```python
from build123d import *

# Parameters (mm, degrees)
PAD_DEPTH       = 15
SKETCH001_W     = 60
SKETCH001_H     = 15
PAD001_DEPTH    = 5
SKETCH002_W     = 60
SKETCH002_H     = 15
PAD002_DEPTH    = 5
FILLET_R        = 7
SKETCH003_W     = 3
SKETCH003_H     = 15
PAD003_DEPTH    = 3
CHAMFER_SIZE    = 2
SKETCH004_R     = 3.25
POCKET_DEPTH    = 60.001
POCKET001_DEPTH = 33
FILLET001_R     = 2


with BuildPart() as part:
    # Sketch → Pad (new body)
    with BuildSketch(Plane.XY):
        Polygon((0, 0), (30, 0), (30, 15), (-15, 15), align=None)
    extrude(amount=PAD_DEPTH)

    # Sketch001 (on Face6 of Pad) → Pad001 (join)
    with BuildSketch(Plane.XY.offset(15)):
        with Locations((0, 7.5)):
            Rectangle(SKETCH001_W, SKETCH001_H)
    extrude(amount=PAD001_DEPTH)

    # Sketch002 (on Face4 of Pad001) → Pad002 (join)
    with BuildSketch(Plane(origin=(0, 0, 0), x_dir=(1, 0, 0), z_dir=(0, 0, -1))):
        with Locations((0, -7.5)):
            Rectangle(SKETCH002_W, SKETCH002_H)
    extrude(amount=PAD002_DEPTH)

    # Fillet
    fillet_edges = [part.edges().sort_by_distance(p)[0] for p in [
        (-7.5, 7.5, 0),
        (-7.5, 7.5, 15),
    ]]
    fillet(fillet_edges, radius=FILLET_R)

    # Sketch003 (on Face9 of Fillet) → Pad003 (join)
    with BuildSketch(Plane.XY):
        with Locations((-28.5, 7.5)):
            Rectangle(SKETCH003_W, SKETCH003_H)
    extrude(amount=PAD003_DEPTH)

    # Chamfer
    chamfer_edges = [part.edges().sort_by_distance(p)[0] for p in [
        (-27, 7.5, 3),
    ]]
    chamfer(chamfer_edges, length=CHAMFER_SIZE)

    # Sketch004 (on Face18 of Chamfer) → Pocket (cut, through all)
    with BuildSketch(Plane.YZ.offset(30)):
        with Locations((7.5, 7.5)):
            Circle(SKETCH004_R)
    extrude(amount=-POCKET_DEPTH, mode=Mode.SUBTRACT)

    # Sketch005 (on Face23 of Pocket) → Pocket001 (cut)
    with BuildSketch(Plane(origin=(-30, 0, 0), x_dir=(0, -1, 0), z_dir=(-1, 0, 0))):
        Polygon((-7.5, 13.562178), (-12.75, 10.531089), (-12.75, 4.468911), (-7.5, 1.437822), (-2.25, 4.468911), (-2.25, 10.531089), align=None)
    extrude(amount=-POCKET001_DEPTH, mode=Mode.SUBTRACT)

    # Fillet001
    fillet001_edges = [part.edges().sort_by_distance(p)[0] for p in [
        (30, 7.5, 20),
        (30, 7.5, -5),
        (0, 0, 20),
        (0, 0, -5),
        (0, 15, 20),
        (0, 15, -5),
    ]]
    fillet(fillet001_edges, radius=FILLET001_R)


solid = part.part
```
Here's how the part is built. I have some questions about the finished solid (model axes, mm). A direction names the side the tool comes from. Give positions to 0.01 mm unless a question says otherwise; leave off trailing zeros. Order: outer loops, then holes, each group sorted by start corner. A loop starts at its lowest first (then second) coordinate and runs counter-clockwise, first axis right, second up. Notation, with made-up numbers: (71.5, 89.25) - (95.5, 89.25) arc R34 cw to (95.5, 121.25) - close; hole circle Ø6 at (78.5, 83.25). An arc over 180 degrees is marked (long way). Answer as a JSON object with one key per item and string values. Group by question number.
Item 1: For P1, Ø3, axis at y = 9.5, z = 9, coming from the -X side, with a flat end and sliding along its axis, tell me the tip position at first contact or that it passes through.
Item 2: If we section it at A-A on z = 5.25: Please give me the cut outline in (x, y).
Item 3: If we mould it in two halves opening along Y, with no side actions, what happens to faces 1 (the flat face through (0, 2.25, 7)), 2 (the cylindrical face through (29.43, 7.61, 19.4)), 3 (the flat face through (6, 0, 7)), 4 (the cylindrical face through (0.42, 14.4, 19.43))? For each: pulls with the +Y half, pulls with the -Y half, needs draft (parallel to the pull), parting line crosses it, or undercut.
Item 4: Please list where these lines run through material, in increasing order: probe 1 along Z at (x, y) = (15.5, 7.5); probe 2 along Z at (x, y) = (-15.5, 3.25); probe 3 along Y at (x, z) = (22.5, 10).
Item 5: If we section it at B-B on z = 9.25: Please give me the cut outline in (x, y).
Item 6: Which directions (+Z, -Z, +X, -X, +Y, -Y) give clear straight access to the entire face, cutting with the end or side of a thin tool? Please do faces 5 (the cylindrical face through (-11.9, 7.77, 1.31)), 6 (the flat face through (30, 11, 8)), 7 (the flat face through (-2.7, 5.42, 12.36)), 8 (the flat face through (-27.3, 7.4, 1.3)).
Result set:
{
 "1": {"P1": "x = 3"},
 "2": {"outline": "(-15.31, 15) - (-13.06, 12.75) - (3, 12.75) - (3, 9.85) - (30, 9.85) - (30, 15) - close; (-2.56, 2.25) - (-0.31, 0) - (30, 0) - (30, 5.15) - (3, 5.15) - (3, 2.25) - close"},
 "3": {"face 1": "undercut", "face 2": "needs draft", "face 3": "pulls with the -Y half", "face 4": "pulls with the +Y half"},
 "4": {"probe 1": "-5 to 4.25, 10.75 to 20", "probe 2": "-5 to 0, 15 to 20", "probe 3": "0 to 5.42, 9.58 to 15"},
 "5": {"outline": "(-15.16, 15) - (-12.91, 12.75) - (3, 12.75) - (3, 10.24) - (30, 10.24) - (30, 15) - close; (-2.41, 2.25) - (-0.16, 0) - (30, 0) - (30, 4.76) - (3, 4.76) - (3, 2.25) - close"},
 "6": {"face 5": "-Y", "face 6": "+Z, -Z, +X, +Y, -Y", "face 7": "-X", "face 8": "+Y, -Y"}
}
